Input: part model. Units: mm. Frame: model coordinates. A direction names the side the tool comes from. Round coordinates to 2 decimals unless told otherwise and drop trailing zeros. Write each loop counter-clockwise with the first axis right and the second up, starting at its lowest first coordinate (ties: lowest second). Pieces come first, ordered by that corner, then holes. Notation, with made-up numbers: (-16, 10.5) -> (25, 10.5) arc R7 cw to (25, 14.5) -> close; hole circle Ø11 at (-39, -19.5). An arc over 180 degrees is marked (long way). Write item = value, one per line.
```python
from build123d import *

# Parameters (mm, degrees)
SKETCH1_R           = 127
BOSS_EXTRUDE1_DEPTH = 6.35
SKETCH2_R           = 6.35
BOSS_EXTRUDE2_DEPTH = 12.7
SKETCH3_R           = 5.715
SKETCH3_W           = 50.8
SKETCH3_H           = 3.175
SKETCH3_W_2         = 3.175
SKETCH3_H_2         = 50.8
CUT_EXTRUDE1_DEPTH  = 181.612575697


with BuildPart() as part:
    # Sketch1 → Boss-Extrude1 (new body)
    with BuildSketch(Plane(origin=(0, 0, 0), x_dir=(1, 0, 0), z_dir=(0, 1, 0))):
        with Locations(Location((0, 0, 0), (0, 0, 270))):
            Circle(SKETCH1_R)
    extrude(amount=BOSS_EXTRUDE1_DEPTH)

    # Sketch2 → Boss-Extrude2 (add)
    with BuildSketch(Plane.XZ):
        with Locations(Location((0, -114.3, 0), (0, 0, 90))):
            Circle(SKETCH2_R)
        with Locations(Location((-98.986703653, 57.15, 0), (0, 0, 90))):
            Circle(SKETCH2_R)
        with Locations(Location((98.986703653, 57.15, 0), (0, 0, 90))):
            Circle(SKETCH2_R)
    extrude(amount=BOSS_EXTRUDE2_DEPTH)

    # Sketch3 → Cut-Extrude1 (cut, through all)
    with BuildSketch(Plane(origin=(0, 6.35, 0), x_dir=(1, 0, 0), z_dir=(0, 1, 0))):
        with Locations(Location((101.6, -31.75, 0), (0, 0, 270))):
            Circle(SKETCH3_R)
        with Locations(Location((-31.75, -101.6, 0), (0, 0, 270))):
            Circle(SKETCH3_R)
        with Locations(Location((-101.6, 31.75, 0), (0, 0, 270))):
            Circle(SKETCH3_R)
        with Locations(Location((31.75, 101.6, 0), (0, 0, 270))):
            Circle(SKETCH3_R)
        with Locations(Location((-78.29630657, -72.113181024, 0), (0, 0, 270))):
            Circle(SKETCH3_R)
        with Locations(Location((-23.30369343, 103.863181024, 0), (0, 0, 270))):
            Circle(SKETCH3_R)
        with Locations((-31.75, -84.1375)):
            Rectangle(SKETCH3_W, SKETCH3_H)
        with Locations((84.1375, -31.75)):
            Rectangle(SKETCH3_W_2, SKETCH3_H_2)
        with Locations((-84.1375, 31.75)):
            Rectangle(SKETCH3_W_2, SKETCH3_H_2)
        with Locations((31.75, 84.1375)):
            Rectangle(SKETCH3_W, SKETCH3_H)
        Polygon((-48.361761314, -71.065027739), (-92.355851826, -45.665027739), (-90.768351826, -42.915397082), (-46.774261314, -68.315397082), align=None)
        Polygon((-37.363238686, 77.415027739), (6.630851826, 102.815027739), (8.218351826, 100.065397082), (-35.775738686, 74.665397082), align=None)
    extrude(amount=-CUT_EXTRUDE1_DEPTH, mode=Mode.SUBTRACT)


solid = part.part
```
1) Draft query along Z for faces 4 (the face through (99, -12.7, 57)), 5 (the face through (-13.471, 3.219, -87.543)), 6 (the face through (94.695, -6.261, 52.47)). Return one class per face: +Z half, -Z half, draft (parallel to the pull), parting line (faces both ways), or undercut.
Solutions:
face_4 = draft
face_5 = undercut
face_6 = parting line
2) Cut plane B-B (z = 54). Return the cut outline in (x, y) (3 decimals), and give its area (3 significant figures).
Solutions:
outline = (-114.948, 0) -> (-104.5, 0) -> (-104.5, -12.7) -> (-93.473, -12.7) -> (-93.473, 0) -> (-77.919, 0) -> (-77.919, 6.35) -> (-114.948, 6.35) -> close; (-71.569, 0) -> (82.55, 0) -> (82.55, 6.35) -> (-71.569, 6.35) -> close; (85.725, 0) -> (93.473, 0) -> (93.473, -12.7) -> (104.5, -12.7) -> (104.5, 0) -> (114.948, 0) -> (114.948, 6.35) -> (85.725, 6.35) -> close
area = 1,680 mm^2
3) Cut plane A-A (z = 101.6). Return the cut outline in (x, y) (3 decimals).
Solutions:
outline = (-76.2, 0) -> (-37.465, 0) -> (-37.465, 6.35) -> (-76.2, 6.35) -> close; (-26.035, 0) -> (76.2, 0) -> (76.2, 6.35) -> (-26.035, 6.35) -> close
4) Cut plane C-C (x = 0). Return the cut outline in (y, z).
Solutions:
outline = (-12.7, -120.65) -> (0, -120.65) -> (0, -127) -> (6.35, -127) -> (6.35, -98.99) -> (0, -98.99) -> (0, -107.95) -> (-12.7, -107.95) -> close; (0, -95.32) -> (6.35, -95.32) -> (6.35, 127) -> (0, 127) -> close
5) First-contact query: P1, Ø6, axis at y = -2, z = 35.5, coming from the -X side; P2, Ø1, axis at y = 2, z = 83.5, coming from the -X side; P3, Ø5, axis at y = 4, z = -81.5, coming from the +X side. Flat tips, straight axial feed; report the tip coordinate or a pass-through.
Solutions:
P1 = -122.57
P2 = -96.12
P3 = 99.44
6) Access query for faces 1 (the face through (-105.283, -6.261, 56.323)), 2 (the face through (-99, -12.7, 57)), 3 (the face through (-15.67, 3.22, -89.94)). Directions: +Z, -Z, +X, -X, +Y, -Y. A direction counts if a zero-diameter tool reaches every point of the face in a straight line with its end or side. Return the directions, or none.
Solutions:
face_1 = -Y
face_2 = +Z, -Z, +X, -X, -Y
face_3 = +Y, -Y
7) Line query: L1, parallel to X at y = 3.25, z = -31.75 (3 decimals); L2, parallel to Y at x = -18.5, z = -89; L3, parallel to X at y = 1.5, z = 73. Output: solid intervals per line, ascending. Write a range as from..to.
Solutions:
L1 = -122.967..-107.315, -95.885..-85.725, -82.55..122.967
L2 = 0..6.35
L3 = -103.92..-83.94, -72.65..103.92
8) Cut plane D-D (z = -114.3). Return the cut outline in (x, y), and give its area (3 significant figures).
Solutions:
outline = (-55.36, 0) -> (-6.35, 0) -> (-6.35, -12.7) -> (6.35, -12.7) -> (6.35, 0) -> (55.36, 0) -> (55.36, 6.35) -> (-55.36, 6.35) -> close
area = 864 mm^2
